Could you check a few things on this model? Use its own coordinates, in mm. A direction names the side the tool comes from. Round coordinates to 2 decimals unless told otherwise and drop trailing zeros. Loops run counter-clockwise (first coordinate to the right, second up) from the corner with the lowest first, then second, coordinate; pieces in that order, holes last. Notation, with made-up numbers: (-20, 88) -> (-6, 88) arc R18 cw to (-6, 116) -> close; hole circle Ø1 at (-7.75, 36.25). An arc over 180 degrees is marked (long way). Write each question's results on one line, items separated by ' | '. Start each with the question number.
1) For P1, Ø8, axis at x = 115, y = -2, coming from the +Z side; P2, Ø2.5, axis at y = 0, z = 0, coming from the -X side; P3, Ø5, axis at x = 35.5, z = 13, coming from the -Y side (3 decimals); P4, Ø6, axis at y = 1, z = 5.5, coming from the +X side, each with a flat end and sliding along its axis, tell me the tip position at first contact or that it passes through.
2) Which directions (+Z, -Z, +X, -X, +Y, -Y) give clear straight access to the entire face, cutting with the end or side of a thin tool? Please do faces 4 (the cylindrical face through (176.888, -19.334, -2.539)), 5 (the conical face through (120.732, -11.1, -12.105)), 6 (the cylindrical face through (99.895, 19.524, -4.336)), 7 (the cylindrical face through (56.756, 9.274, -2.059)), 8 (the cylindrical face through (86.5, -7.7, -0.1)).
3) Imagine slicing it at B-B, the plane x = 151. List the corners of the cut face in (y, z) for me.
4) Imagine slicing it at C-C, the plane x = 110. List the corners of the cut face in (y, z) for me.
5) If I drill on probe 1 along Y at (x, z) = (177.15, 0); probe 2 along Z at (x, y) = (181, 0); probe 3 along X at (y, z) = (3.5, -6), over which ranges is the centre line in solid material (lowest first)?
6) Imagine slicing it at A-A, the plane x = 51.5. List the corners of the cut face in (y, z) for me, plus the area to 3 significant figures.
7) We'd pull the mould along Z, two halves only. Please class faces 1 (the cylindrical face through (46.5, -7.7, 0.1)), 2 (the cylindrical face through (20.73, -0.38, -8.59)), 3 (the flat face through (22, -8.5, -2.2)): pulls with the +Z half, pulls with the -Z half, needs draft (parallel to the pull), parting line crosses it, or undercut.
from build123d import *

# Parameters (mm, degrees)
F3_START             = 6
F3_DEPTH             = 9.4
F4_R                 = 13
F5_DEPTH             = 6
F8_D                 = 2
F8_DEPTH             = 6.3
F8_CSINK_D           = 3
F8_CSINK_ANGLE       = 90
F8_TIP               = 0.600860619
F8_ON_F6_D           = 2
F8_ON_F6_DEPTH       = 6.3
F8_ON_F6_CSINK_D     = 3
F8_ON_F6_CSINK_ANGLE = 90
F8_ON_F6_TIP         = 0.600860619


with BuildPart() as f1:
    # F0 (on Front) → F1 (revolve)
    with BuildSketch(Plane.XZ):
        Polygon((1, 8.5), (0, 7.5), (0, 0), (169, 0), (169, 15), (126, 15), (107.5, 20), (92.5, 20), (92.5, 9.5), (22, 9.5), (22, 8.6), (19.5, 8.6), (19.5, 8.5), align=None)
        Polygon((169, 15), (169, 0), (185, 0), (185, 19.5), (169, 19.5), align=None)
    revolve(axis=Axis((105.2958741784, 0, 0), (1, 0, 0)))

    # F2 (on Front) → F3 (cut)
    with BuildSketch(Plane.XZ.offset(F3_START)):
        with BuildLine():
            ThreePointArc((83.5, -3), (86.5, 0), (83.5, 3))
            Line((83.5, 3), (49.5, 3))
            ThreePointArc((49.5, 3), (46.5, 0), (49.5, -3))
            Line((49.5, -3), (83.5, -3))
        make_face()
    extrude(amount=F3_DEPTH, mode=Mode.SUBTRACT)

    # F4 (on face) → F5 (cut)
    with BuildSketch(Plane.YZ.offset(185)):
        Circle(F4_R)
    extrude(amount=-F5_DEPTH, mode=Mode.SUBTRACT)

    # F8
    with Locations(Plane(origin=(0, 0, 0), x_dir=(0, -1, 0), z_dir=(-1, 0, 0))):
        with Locations((0, 0)):
            CounterSinkHole(F8_D / 2, F8_CSINK_D / 2, depth=F8_DEPTH, counter_sink_angle=F8_CSINK_ANGLE)
            with Locations((0, 0, -(F8_DEPTH + F8_TIP / 2))):  # 118° drill point
                Cone(0, F8_D / 2, F8_TIP, mode=Mode.SUBTRACT)

    # F8 on F6
    with Locations(Plane.YZ.offset(179)):
        with Locations((0, 0)):
            CounterSinkHole(F8_ON_F6_D / 2, F8_ON_F6_CSINK_D / 2, depth=F8_ON_F6_DEPTH, counter_sink_angle=F8_ON_F6_CSINK_ANGLE)
            with Locations((0, 0, -(F8_ON_F6_DEPTH + F8_ON_F6_TIP / 2))):  # 118° drill point
                Cone(0, F8_ON_F6_D / 2, F8_ON_F6_TIP, mode=Mode.SUBTRACT)


solid = f1.part
Checked values:
1) P1: z = 18.99 | P2: x = 0.25 | P3: through | P4: x = 179
2) face 4: +X | face 5: none | face 6: +X, -X | face 7: -X | face 8: -Y
3) outline: circle Ø30 at (0, 0)
4) outline: circle Ø38.65 at (0, 0)
5) probe 1: -19.5 to -1, 1 to 19.5 | probe 2: -19.5 to -13, 13 to 19.5 | probe 3: 0 to 179
6) outline: (-9.01, -3) arc R9.5 ccw (long way) to (-9.01, 3) -> (-6, 3) -> (-6, -3) -> close | area: 263 mm^2
7) face 1: undercut | face 2: parting line crosses it | face 3: needs draft
